from build123d import *

# Parameters (mm, degrees)
SKETCH1_R                = 6.25
BOSS_EXTRUDE1_DEPTH      = 37
BOSS_EXTRUDE1_DEPTH_BACK = 45
SKETCH4_W                = 6
SKETCH4_H                = 4.5
CUT_EXTRUDE1_DEPTH       = 13
BOSS_EXTRUDE2_DEPTH      = 46
FILLET1_R                = 3


with BuildPart() as part:
    # Sketch1 → Boss-Extrude1 (new body, two sides)
    with BuildSketch(Plane.XY) as boss_extrude1_sk:
        Circle(SKETCH1_R)
    extrude(amount=BOSS_EXTRUDE1_DEPTH)
    extrude(boss_extrude1_sk.sketch, amount=-BOSS_EXTRUDE1_DEPTH_BACK)

    # Sketch4 → Cut-Extrude1 (cut)
    with BuildSketch(Plane(origin=(0, 0, -45), x_dir=(-1, 0, 0), z_dir=(0, 0, -1))):
        with Locations((0, 6.25)):
            Rectangle(SKETCH4_W, SKETCH4_H)
    extrude(amount=-CUT_EXTRUDE1_DEPTH, mode=Mode.SUBTRACT)

    # Sketch5 → Boss-Extrude2 (add)
    with BuildSketch(Plane.XY.offset(-23)):
        Polygon((3.732897661, 6.176472163), (-3.482532969, 6.321020286), (-7.21543063, 0.144548123), (-3.732897661, -6.176472163), (3.482532969, -6.321020286), (7.21543063, -0.144548123), align=None)
    extrude(amount=BOSS_EXTRUDE2_DEPTH)

    # Fillet1
    fillet1_edges = [part.edges().sort_by_distance(p)[0] for p in [
        (7.21543063, -0.144548123, 0),
        (3.732897661, 6.176472163, 0),
        (-3.482532969, 6.321020286, 0),
        (-7.21543063, 0.144548123, 0),
        (-3.732897661, -6.176472163, 0),
        (3.482532969, -6.321020286, 0),
    ]]
    fillet(fillet1_edges, radius=FILLET1_R)


solid = part.part
Here's how the part is built. I have some questions about the finished solid (model axes, mm). A direction names the side the tool comes from. Coordinates: 2 decimals unless noted, no trailing zeros. Write each loop counter-clockwise with the first axis right and the second up, starting at its lowest first coordinate (ties: lowest second). Pieces come first, ordered by that corner, then holes.
1) I'm going to push flat-ended pins straight in: pin 1 (4 mm diameter, centred on x = -1.5, z = -1.5, fed in from +Y); pin 2 (0.9 mm diameter, centred on x = 4, y = -5.5, fed in from +Z); pin 3 (3 mm diameter, centred on x = -5, z = -26, fed in from +Y); pin 4 (0.7 mm diameter, centred on x = -6.5, y = 1.5, fed in from -Z). Where does each tip first touch, or does it pass through?
Filled in:
pin 1: stops at y = 6.29
pin 2: stops at z = 23
pin 3: stops at y = 5.18
pin 4: stops at z = -23
2) If we section it at A-A (z = 24): List the corners of the cut face in (x, y) for me, plus the area to 3 significant figures.
Filled in:
outline: circle Ø12.5 at (0, 0)
area: 123 mm2
3) Thinking about a two-plate mould opening in X: for faces 1 (the face through (-5.335, 3.255, -0.322)), 2 (the face through (0, 4, -39)), 3 (the face through (6.4, -0.1, -23)), which applies, +X half, -X half, draft (parallel to the pull), parting line (faces both ways), or undercut?
Filled in:
face 1: -X half
face 2: undercut
face 3: draft
4) If I drill on line 1 (Y direction, x = -2, z = -18.5); line 2 (Y direction, x = 1, z = -0.5); line 3 (X direction, y = -3, z = 10), over which ranges is the centre line in solid material (lowest first)?
Filled in:
line 1: y = -6.21 to 6.28
line 2: y = -6.27 to 6.23
line 3: x = -5.48 to 5.49
5) Which directions (+Z, -Z, +X, -X, +Y, -Y) give clear straight access to the entire face, cutting with the end or side of a thin tool? Please do faces 4 (the face through (-3.2, -5.6, 23)), 5 (the face through (-3, 5, -39)), 6 (the face through (3.4, 5.5, 23)), 7 (the face through (-3, 5.7, 23)).
Filled in:
face 4: +Z, -X, -Y
face 5: -Z, +Y
face 6: +Z, +X, +Y
face 7: +Z, -X, +Y
6) If we section it at B-B (y = 0): List the corners of the cut face in (x, z) for me.
Filled in:
outline: (-6.75, -23) - (-6.25, -23) - (-6.25, -45) - (6.25, -45) - (6.25, -23) - (6.75, -23) - (6.75, 23) - (6.25, 23) - (6.25, 37) - (-6.25, 37) - (-6.25, 23) - (-6.75, 23) - close
7) If we section it at C-C (z = -38): List the corners of the cut face in (x, y) for me, plus the area to 3 significant figures.
Filled in:
outline: (-3, 4) - (-3, 5.48) arc R6.25 ccw (long way) to (3, 5.48) - (3, 4) - close
area: 111 mm2
